Model file for the job. Use its own axes, mm. Give positions to 0.01 mm unless a question says otherwise; leave off trailing zeros. Loops run counter-clockwise (first coordinate to the right, second up) from the corner with the lowest first, then second, coordinate; pieces in that order, holes last. Notation, with made-up numbers: (20.25, 42.5) -> (71.25, 42.5) arc R23 ccw to (71.25, 50.5) -> close; hole circle Ø2 at (71, -22.5). An arc over 180 degrees is marked (long way). Use CSV: the item, a comma, the result in double quotes. Start each with the question number.
(1) Cut at D-D on z = -9.5. Write the cut outline in (x, y) (3 decimals), then the cut area to 3 significant figures.
(2) Flat gauge pins, fed straight in: pin 1 (1 mm diameter, centred on y = 1.5, z = 8, fed in from -X); pin 2 (2 mm diameter, centred on x = 13.5, y = 1.5, fed in from -Z); pin 3 (1.5 mm diameter, centred on y = 2, z = -6, fed in from +X); pin 4 (1.3 mm diameter, centred on x = -10, y = 2.5, fed in from +Z). Where does each tip first touch, or does it go through?
(3) Cut at C-C on y = 1.2. Write the cut outline in (x, z).
(4) Drill centre lines: probe 1 along Z at (x, y) = (3, 2.25); probe 2 along Y at (x, z) = (-16.5, 18); probe 3 along Y at (x, z) = (19, 15). Where is each one in solid material? Low to high.
(5) Cut at A-A on z = -20. Write the cut outline in (x, y).
from build123d import *

# Parameters (mm, degrees)
BOSS_EXTRU_1_DEPTH         = 0.6
ESQUISSE3_W                = 48.088583049
ESQUISSE3_H                = 40.702531731
BOSS_EXTRU_2_DEPTH         = 3
CONG_1_R                   = 0.4
ESQUISSE4_W                = 47.99
ESQUISSE4_H                = 27.83
BOSS_EXTRU_3_DEPTH         = 0.1
ESQUISSE5_R                = 0.381
ENL_V_MAT_EXTRU_1_DEPTH    = 38.55059167
R_P_TITION_LIN_AIRE1_COUNT = 20
R_P_TITION_LIN_AIRE1_PITCH = 2.54
ESQUISSE7_R                = 0.381
ENL_V_MAT_EXTRU_3_DEPTH    = 38.435332241
R_P_TITION_LIN_AIRE2_COUNT = 3
R_P_TITION_LIN_AIRE2_PITCH = 2.54
ESQUISSE9_R                = 0.381
ENL_V_MAT_EXTRU_4_DEPTH    = 38.435332241
R_P_TITION_LIN_AIRE3_COUNT = 3
R_P_TITION_LIN_AIRE3_PITCH = 2.54


with BuildPart() as part:
    # cadre ecran → Boss.-Extru.1 (new body)
    with BuildSketch(Plane(origin=(0, 0, 0), x_dir=(1, 0, 0), z_dir=(0, 1, 0))):
        Polygon((0, -20.787329411), (27.5, -20.787329411), (27.5, 25.21), (-27.5, 25.21), (-27.5, -20.787329411), align=None)
    extrude(amount=BOSS_EXTRU_1_DEPTH)

    # Esquisse3 → Boss.-Extru.2 (add)
    with BuildSketch(Plane(origin=(0, 0.6, 0), x_dir=(1, 0, 0), z_dir=(0, 1, 0))):
        with Locations((0.023851228, 2.523244052)):
            Rectangle(ESQUISSE3_W, ESQUISSE3_H)
    extrude(amount=BOSS_EXTRU_2_DEPTH)

    # Congé1
    cong_1_edges = [part.edges().sort_by_distance(p)[0] for p in [
        (0.023851228, 3.6, 17.828021814),
        (0.023851228, 3.6, -22.874509917),
    ]]
    fillet(cong_1_edges, radius=CONG_1_R)

    # Esquisse4 → Boss.-Extru.3 (add)
    with BuildSketch(Plane(origin=(0, 3.6, 0), x_dir=(1, 0, 0), z_dir=(0, 1, 0))):
        Rectangle(ESQUISSE4_W, ESQUISSE4_H)
    extrude(amount=BOSS_EXTRU_3_DEPTH)

    # Esquisse5 → Enlèv. mat.-Extru.1 (cut, through all)
    with BuildSketch(Plane(origin=(-0.148451016, 0.6, 0.009042233), x_dir=(1, 0, 0), z_dir=(0, 1, 0))):
        with Locations(Location((-23.976340586, 23.783183719, 0), (0, 0, 270))):
            Circle(ESQUISSE5_R)
    enl_v_mat_extru_1 = extrude(amount=-ENL_V_MAT_EXTRU_1_DEPTH, mode=Mode.SUBTRACT)

    # Répétition linéaire1: Enlèv. mat.-Extru.1 ×20
    with Locations(*[(i * R_P_TITION_LIN_AIRE1_PITCH, 0, 0) for i in range(1, R_P_TITION_LIN_AIRE1_COUNT)]):
        add(enl_v_mat_extru_1, mode=Mode.SUBTRACT)

    # Esquisse7 → Enlèv. mat.-Extru.3 (cut, through all)
    with BuildSketch(Plane(origin=(0, 0.6, 0), x_dir=(1, 0, 0), z_dir=(0, 1, 0))):
        with Locations(Location((-24.124791601, -19.380242651, 0), (0, 0, 270))):
            Circle(ESQUISSE7_R)
    enl_v_mat_extru_3 = extrude(amount=-ENL_V_MAT_EXTRU_3_DEPTH, mode=Mode.SUBTRACT)

    # Répétition linéaire2: Enlèv. mat.-Extru.3 ×3
    with Locations(*[(i * R_P_TITION_LIN_AIRE2_PITCH, 0, 0) for i in range(1, R_P_TITION_LIN_AIRE2_COUNT)]):
        add(enl_v_mat_extru_3, mode=Mode.SUBTRACT)

    # Esquisse9 → Enlèv. mat.-Extru.4 (cut, through all)
    with BuildSketch(Plane(origin=(0, 0.6, 0), x_dir=(1, 0, 0), z_dir=(0, 1, 0))):
        with Locations(Location((24.135208399, -19.380242651, 0), (0, 0, 270))):
            Circle(ESQUISSE9_R)
    enl_v_mat_extru_4 = extrude(amount=-ENL_V_MAT_EXTRU_4_DEPTH, mode=Mode.SUBTRACT)

    # Répétition linéaire3: Enlèv. mat.-Extru.4 ×3
    with Locations(*[(-i * R_P_TITION_LIN_AIRE3_PITCH, 0, 0) for i in range(1, R_P_TITION_LIN_AIRE3_COUNT)]):
        add(enl_v_mat_extru_4, mode=Mode.SUBTRACT)


solid = part.part
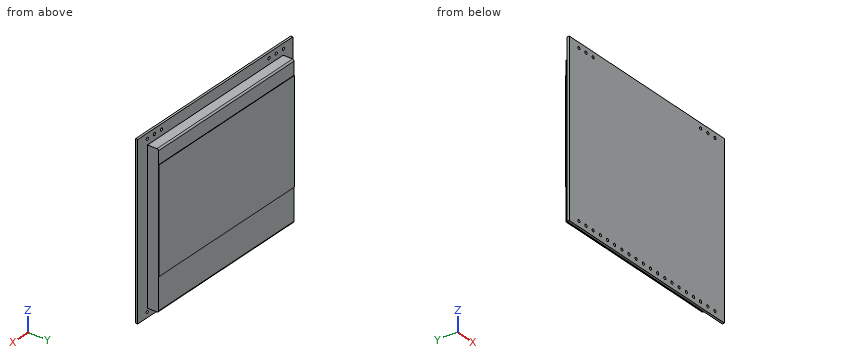
Check result:
1,outline,"(-27.5, 0) -> (27.5, 0) -> (27.5, 0.6) -> (24.068, 0.6) -> (24.068, 3.6) -> (23.995, 3.6) -> (23.995, 3.7) -> (-23.995, 3.7) -> (-23.995, 3.6) -> (-24.02, 3.6) -> (-24.02, 0.6) -> (-27.5, 0.6) -> close"
1,area,"182 mm²"
2,pin 1,"x = -24.02"
2,pin 2,"z = -25.21"
2,pin 3,"x = 24.07"
2,pin 4,"z = 17.83"
3,outline,"(-24.02, -22.87) -> (24.07, -22.87) -> (24.07, 17.83) -> (-24.02, 17.83) -> close"
4,probe 1,"-22.87 to 17.83"
4,probe 2,"0 to 0.6"
4,probe 3,"0 to 3.6"
5,outline,"(-27.5, 0) -> (27.5, 0) -> (27.5, 0.6) -> (24.07, 0.6) -> (24.07, 3.6) -> (-24.02, 3.6) -> (-24.02, 0.6) -> (-27.5, 0.6) -> close"
